Autodesk Inventor part; units mm, degrees
ref_plane "YZ Plane" through (0, 0, 0) normal (1, 0, 0) x (0, 1, 0)
ref_plane "XZ Plane" through (0, 0, 0) normal (0, 1, 0) x (-1, 0, 0)
ref_plane "XY Plane" through (0, 0, 0) normal (0, 0, 1) x (1, 0, 0)
sketch "Sketch1" plane through (0, 0, 0) normal (0, 0, 1) x (1, 0, 0)
  circle A0 centre (0, 0) radius 8.255
  circle A1 centre (0, 0) radius 2.9845
  line L0 (-8.2498, 0.2936) -> (-2.9768, 0.2936)
  line L1 (-2.9768, 0.2936) -> (-2.9768, -0.2144)
  line L2 (-2.9768, -0.2144) -> (-8.2498, -0.2144)
  line L3 (-8.1951, 0.2936) -> (-8.1951, -0.2144)
  line L4 (0, 8.255) -> (0, -8.255) construction
  line L5 (8.2498, 0.2936) -> (2.9768, 0.2936)
  line L6 (2.9768, 0.2936) -> (2.9768, -0.2144)
  line L7 (2.9768, -0.2144) -> (8.2498, -0.2144)
  line L8 (8.1951, 0.2936) -> (8.1951, -0.2144)
  dimension "d13" = 5.969
  dimension "d0" = 16.51
  dimension "d14" = 0.508
extrude "Extrusion1" add sketch "Sketch1" along normal blind 9.3726
shell "Shell1" thickness 0.381 removed faces 1 at (-0.9758, 3.8899, 0)
extrude "Extrusion3" cut sketch "Sketch1" along normal blind 17.526 contours L0 L1 A1 L2 L3 | L1 A1
extrude "Extrusion4" cut sketch "Sketch1" along normal blind 17.526 contours L6 A1 L1 | A1 L6 | L1 A1
extrude "Extrusion5" cut sketch "Sketch1" along normal blind 17.526 contours L8 L7 A1 L6 L5 | A1 L6
sketch "Sketch2" plane through (0, 0, 9.3726) normal (0, 0, 1) x (1, 0, 0)
  circle A0 centre (0, 0) radius 8.255
  line L0 (0, 8.255) -> (0, -8.255)
  line L1 (8.1951, -0.2144) -> (2.9768, -0.2144)
  line L2 (8.1951, -0.2144) -> (-8.3257, -0.2144)
properties part number "dis1"
Here's how the part is built. I have some questions about the finished solid (model axes, mm). A direction names the side the tool comes from. Coordinates: 2 decimals unless noted, no trailing zeros. Order: outer loops, then holes, each group sorted by start corner. A loop starts at its lowest first (then second) coordinate and runs counter-clockwise, first axis right, second up. Notation, with made-up numbers: (-28, -7.5) - (18, -7.5) arc R33 ccw to (18, 27.5) - close; hole circle Ø10 at (84.5, 39.25). An arc over 180 degrees is marked (long way). One line per question, with ' | ' between items.
(1) Suppose I cut it at A-A on y = 0. List the corners of the cut face in (x, z) for me (3 decimals), and give its area (3 significant figures).
Report:
outline: (-8.255, 0) - (-8.195, 0) - (-8.195, 9.373) - (-8.255, 9.373) - close; (8.195, 0) - (8.255, 0) - (8.255, 9.373) - (8.195, 9.373) - close | area: 1.12 mm2
(2) If I drill on L1, parallel to Z at x = 4.75, y = 3.5; L2, parallel to X at y = 5.75, z = 5; L3, parallel to Y at x = 3.5, z = 5.5, over which ranges is the centre line in solid material (lowest first)?
Report:
L1: z = 8.99 to 9.37 | L2: x = -5.92 to -5.38, 5.38 to 5.92 | L3: y = -7.48 to -7.05, 7.05 to 7.48
(3) If we mould it in two halves opening along Y, with no side actions, what happens to faces 1 (the flat face through (0, -4, 9.373)), 2 (the flat face through (0, 4, 8.992)), 3 (the cylindrical face through (7.874, -2.48, 4.621))? For each: pulls with the +Y half, pulls with the -Y half, needs draft (parallel to the pull), parting line crosses it, or undercut.
Report:
face 1: needs draft | face 2: undercut | face 3: parting line crosses it
(4) Suppose I cut it at C-C on x = 2.75. List the corners of the cut face in (y, z) for me, and give its area (3 significant figures).
Report:
outline: (-7.78, 0) - (-7.38, 0) - (-7.38, 8.99) - (-1.16, 8.99) - (-1.16, 9.37) - (-7.78, 9.37) - close; (1.16, 8.99) - (7.38, 8.99) - (7.38, 0) - (7.78, 0) - (7.78, 9.37) - (1.16, 9.37) - close | area: 12.3 mm2
(5) For faces 4 (the cylindrical face through (-0.063, 2.984, 9.179)), 5 (the flat face through (4, -7, 0)), 6 (the flat face through (0, -4, 8.992)), which set-ups out of +Z, -Z, +X, -X, +Y, -Y let a thin tool reach every point of the face, with its end or its side?
Report:
face 4: +Z, -Z | face 5: -Z, +X, -X, +Y, -Y | face 6: -Z
(6) Suppose I cut it at D-D on y = 5.75. List the corners of the cut face in (x, z) for me, and give its area (3 significant figures).
Report:
outline: (-5.92, 0) - (-5.38, 0) - (-5.38, 8.99) - (5.38, 8.99) - (5.38, 0) - (5.92, 0) - (5.92, 9.37) - (-5.92, 9.37) - close | area: 14.3 mm2
(7) Will these pins go through, and if not, where does the flat tip stop? pin 1 (4 mm diameter, centred on x = -5.5, z = 3, fed in from +Y); pin 2 (4 mm diameter, centred on x = -4, y = -3, fed in from -Z); pin 3 (3 mm diameter, centred on y = 5, z = 6.5, fed in from -X).
Report:
pin 1: stops at y = 7.48 | pin 2: stops at z = 8.99 | pin 3: stops at x = -7.48
(8) Suppose I cut it at B-B on z = 3.25. List the corners of the cut face in (x, y) for me (3 decimals), and give its area (3 significant figures).
Report:
outline: circle Ø16.51 at (0, 0); hole (-8.195, -0.214) - (-7.871, -0.214) arc R7.874 ccw to (7.871, -0.214) - (8.195, -0.214) - (8.195, 0.294) - (7.869, 0.294) arc R7.874 ccw to (-7.869, 0.294) - (-8.195, 0.294) - close | area: 19.0 mm2
